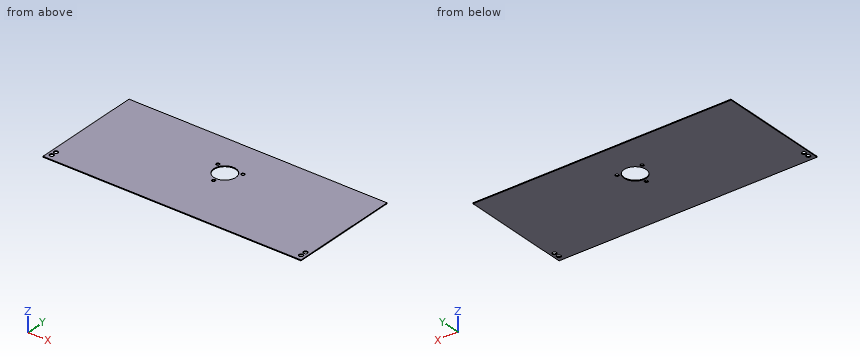
```python
from build123d import *

# Parameters (mm, degrees)
BOSS_EXTRUDE2_DEPTH            = 1
F_5_0MM_DOWEL_HOLE4_AT_2_COUNT = 2
F_5_0MM_DOWEL_HOLE4_AT_2_PITCH = 6.666666667
F_5_0MM_DOWEL_HOLE4_AT_3_COUNT = 2
F_5_0MM_DOWEL_HOLE4_AT_3_PITCH = 294.8
F_5_0MM_DOWEL_HOLE4_AT_4_COUNT = 2
F_5_0MM_DOWEL_HOLE4_AT_4_PITCH = 294.875371037
F_4_0MM_DOWEL_HOLE1_AT_2_COUNT = 2
F_4_0MM_DOWEL_HOLE1_AT_2_PITCH = 29.641373273
F_4_0MM_DOWEL_HOLE1_AT_3_COUNT = 2
F_4_0MM_DOWEL_HOLE1_AT_3_PITCH = 29.619508559
SKETCH14_R                     = 13.01
CUT_EXTRUDE1_DEPTH             = 10
BOSS_EXTRUDE4_DEPTH            = 1


with BuildPart() as part:
    # Sketch1 → Boss-Extrude2 (new body)
    with BuildSketch(Plane.XY):
        with BuildLine():
            Line((-152.4, -80.25), (152.4, -80.25))
            Line((152.4, -80.25), (152.4, -60.25))
            ThreePointArc((152.4, -60.25), (0, 50.334231889), (-152.4, -60.25))
            Line((-152.4, -60.25), (-152.4, -80.25))
        make_face()
    extrude(amount=BOSS_EXTRUDE2_DEPTH)

    # Sketch9 → Ø5.0mm Dowel Hole4 (revolve, cut)
    with BuildSketch(Plane(origin=(-147.4, -66.916666667, 1), x_dir=(0, -1, 0), z_dir=(1, 0, 0))):
        Polygon((0, 0), (0, 2.502151548), (2.5, 1), (2.5, 0.025), (2.525, 0), align=None)
    f_5_0mm_dowel_hole4 = revolve(axis=Axis((-147.4, -66.916666667, 7.35), (0, 0, -1)), mode=Mode.SUBTRACT)

    # Ø5.0mm Dowel Hole4 at 2: Ø5.0mm Dowel Hole4 ×2
    with Locations(*[(0, -i * F_5_0MM_DOWEL_HOLE4_AT_2_PITCH, 0) for i in range(1, F_5_0MM_DOWEL_HOLE4_AT_2_COUNT)]):
        add(f_5_0mm_dowel_hole4, mode=Mode.SUBTRACT)

    # Ø5.0mm Dowel Hole4 at 3: Ø5.0mm Dowel Hole4 ×2
    with Locations(*[(i * F_5_0MM_DOWEL_HOLE4_AT_3_PITCH, 0, 0) for i in range(1, F_5_0MM_DOWEL_HOLE4_AT_3_COUNT)]):
        add(f_5_0mm_dowel_hole4, mode=Mode.SUBTRACT)

    # Ø5.0mm Dowel Hole4 at 4: Ø5.0mm Dowel Hole4 ×2
    with Locations(*[Vector(0.9997443969730838, -0.02260842146026871, 0) * (i * F_5_0MM_DOWEL_HOLE4_AT_4_PITCH) for i in range(1, F_5_0MM_DOWEL_HOLE4_AT_4_COUNT)]):
        add(f_5_0mm_dowel_hole4, mode=Mode.SUBTRACT)

    # Sketch13 → Ø4.0mm Dowel Hole1 (revolve, cut)
    with BuildSketch(Plane(origin=(-14.91881086, 8.587973147, 0), x_dir=(0, 1, 0), z_dir=(1, 0, 0))):
        Polygon((0, 0), (0, 1), (2, 1), (2, 0.025), (2.025, 0), align=None)
    f_4_0mm_dowel_hole1 = revolve(axis=Axis((-14.91881086, 8.587973147, -6.35), (0, 0, 1)), mode=Mode.SUBTRACT)

    # Ø4.0mm Dowel Hole1 at 2: Ø4.0mm Dowel Hole1 ×2
    with Locations(*[Vector(0.9999955957234619, -0.0029679173975410726, 0) * (i * F_4_0MM_DOWEL_HOLE1_AT_2_PITCH) for i in range(1, F_4_0MM_DOWEL_HOLE1_AT_2_COUNT)]):
        add(f_4_0mm_dowel_hole1, mode=Mode.SUBTRACT)

    # Ø4.0mm Dowel Hole1 at 3: Ø4.0mm Dowel Hole1 ×2
    with Locations(*[Vector(0.5036819172784638, -0.8638891863003557, 0) * (i * F_4_0MM_DOWEL_HOLE1_AT_3_PITCH) for i in range(1, F_4_0MM_DOWEL_HOLE1_AT_3_COUNT)]):
        add(f_4_0mm_dowel_hole1, mode=Mode.SUBTRACT)

    # Sketch14 → Cut-Extrude1 (cut)
    with BuildSketch(Plane(origin=(0, 0, 0), x_dir=(-1, 0, 0), z_dir=(0, 0, -1))):
        Circle(SKETCH14_R)
    extrude(amount=-CUT_EXTRUDE1_DEPTH, mode=Mode.SUBTRACT)

    # Sketch15 → Boss-Extrude4 (add)
    with BuildSketch(Plane(origin=(0, 0, 0), x_dir=(-1, 0, 0), z_dir=(0, 0, -1))):
        with BuildLine():
            ThreePointArc((-152.4, -60.25), (0, 40.202429788), (152.4, -60.25))
            ThreePointArc((152.4, -60.25), (0, 50.334231889), (-152.4, -60.25))
        make_face()
        with BuildLine():
            Line((-152.4, 50.334231889), (-152.4, -60.25))
            ThreePointArc((-152.4, -60.25), (-94.147002198, 19.775508453), (8.24e-07, 50.334231889))
            Line((8.24e-07, 50.334231889), (-152.4, 50.334231889))
        make_face()
        with BuildLine():
            ThreePointArc((8.24e-07, 50.334231889), (94.147002865, 19.775507969), (152.4, -60.25))
            Line((152.4, -60.25), (152.4, 50.334231889))
            Line((152.4, 50.334231889), (8.24e-07, 50.334231889))
        make_face()
    extrude(amount=-BOSS_EXTRUDE4_DEPTH)


solid = part.part
```
Verification items for the finished model (mm, model axes). Give positions to 0.01 mm unless a question says otherwise; leave off trailing zeros. Loops run counter-clockwise (first coordinate to the right, second up) from the corner with the lowest first, then second, coordinate; pieces in that order, holes last. Notation, with made-up numbers: M -17,10.25 L 18,10.25 A19 cw 18,20.25 Z; hole C 21,61.25 d11. An arc over 180 degrees is marked long. One line per question, with ' | ' between items.
Item 1: Thickness scan on line 1 (Y direction, x = -147.4, z = 0.4); line 2 (X direction, y = 10, z = 0.1); line 3 (X direction, y = -17, z = 0.7). Record the ranges inside material, lowest first. Write a range as [from, to].
Completed:
line 1: y = [-80.25, -76.08], [-71.08, -69.42], [-64.42, 50.33] | line 2: x = [-152.4, -16.34], [-13.5, -8.32], [8.32, 13.4], [16.05, 152.4] | line 3: x = [-152.4, -2], [2, 152.4]
Item 2: Section check B-B, the plane z = 0.25. State how many separate pieces and enclosed holes the cut face has, plus the area to 3 significant figures.
Completed:
separate pieces: 1 | enclosed holes: 8 | area: 39,200 mm^2
Item 3: Section check A-A, the plane y = 0. Record the cut outline in (x, z), plus the area to 3 significant figures.
Completed:
outline: M -152.4,0 L -13.01,0 L -13.01,1 L -152.4,1 Z; M 13.01,0 L 152.4,0 L 152.4,1 L 13.01,1 Z | area: 279 mm^2
